```python
from build123d import *

# Parameters (mm, degrees)
BOSS_EXTRUDE1_DEPTH = 18.5


with BuildPart() as part:
    # Sketch1 → Boss-Extrude1 (new body)
    with BuildSketch(Plane.YZ):
        with BuildLine():
            Line((-4.326661531, 9.95), (4.326661531, 9.95))
            ThreePointArc((4.326661531, 9.95), (7.672108576, 7.672108576), (9.95, 4.326661531))
            Line((9.95, 4.326661531), (9.95, -4.326661531))
            ThreePointArc((9.95, -4.326661531), (7.672108576, -7.672108576), (4.326661531, -9.95))
            Line((4.326661531, -9.95), (-4.326661531, -9.95))
            ThreePointArc((-4.326661531, -9.95), (-7.672108576, -7.672108576), (-9.95, -4.326661531))
            Line((-9.95, -4.326661531), (-9.95, 4.326661531))
            ThreePointArc((-9.95, 4.326661531), (-7.672108576, 7.672108576), (-4.326661531, 9.95))
        make_face()
    extrude(amount=BOSS_EXTRUDE1_DEPTH)


solid = part.part
```
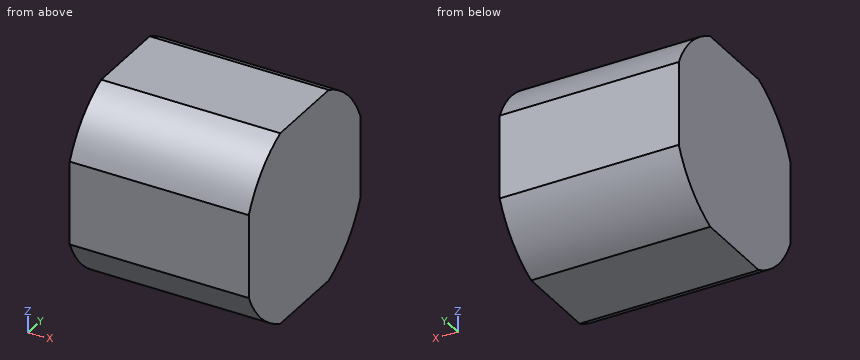
Model file for the job. Use its own axes, mm. Give positions to 0.01 mm unless a question says otherwise; leave off trailing zeros. Write each loop counter-clockwise with the first axis right and the second up, starting at its lowest first coordinate (ties: lowest second). Pieces come first, ordered by that corner, then holes. Notation, with made-up numbers: (-19, -34.75) - (15, -34.75) arc R29 ccw to (15, 1.25) - close; hole circle Ø5 at (-14, 35). An arc over 180 degrees is marked (long way). One line per question, with ' | ' between items. Start each with the question number.
(1) Pin check, flat tip, straight feed: P1, Ø3, axis at x = 4.5, y = -6, coming from the +Z side. Stop position of the tip, or through.
(2) Wall check: line 1 along Z through (x, y) = (14, 6.75); line 2 along Z through (x, y) = (15.5, -5.5); line 3 along Y through (x, z) = (9.25, -8.25). Give the ranges that are in metal, low to high. Write a range as from..to.
(3) Slice it at C-C on y = 6.75. Write the cut outline in (x, z).
(4) Slice it at A-A on x = 4.5. Write the cut outline in (y, z).
(5) Slice it at B-B on z = 4.75. Write the cut outline in (x, y) (3 decimals).
Results below:
1) P1: z = 9.87
2) line 1: -8.49..8.49 | line 2: -9.35..9.35 | line 3: -7.05..7.05
3) outline: (0, -8.49) - (18.5, -8.49) - (18.5, 8.49) - (0, 8.49) - close
4) outline: (-9.95, -4.33) arc R10.85 ccw to (-4.33, -9.95) - (4.33, -9.95) arc R10.85 ccw to (9.95, -4.33) - (9.95, 4.33) arc R10.85 ccw to (4.33, 9.95) - (-4.33, 9.95) arc R10.85 ccw to (-9.95, 4.33) - close
5) outline: (0, -9.755) - (18.5, -9.755) - (18.5, 9.755) - (0, 9.755) - close
